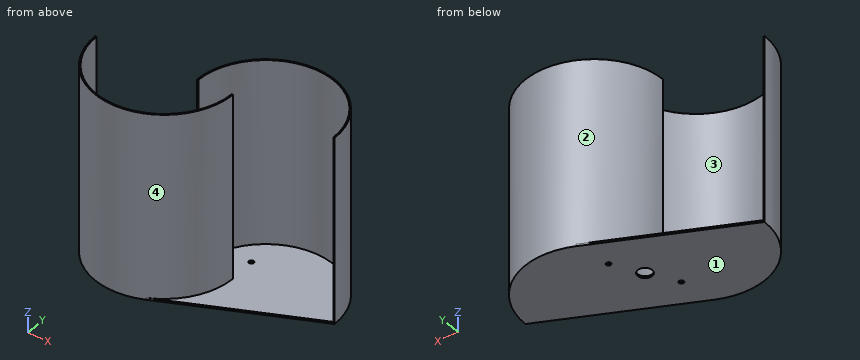
Autodesk Fusion 360 part; units mm, degrees
sketch "Turbine" plane through (0, 0, 0) normal (0, 0, 1) x (1, 0, 0) in component "Savonius Turbine"
  line L0 (10.5, 0) -> (-10.5, 0) construction
  arc A0 (74.2, 0) -> (-10.5, 0) centre (31.85, 0) ccw
  line L1 (31.85, 0) -> (74.2, 0) construction
  line L2 (31.85, 0) -> (-10.5, 0) construction
  arc A1 (-74.2, 0) -> (10.5, 0) centre (-31.85, 0) ccw
  line L3 (-31.85, 0) -> (-74.2, 0) construction
  line L4 (-31.85, 0) -> (10.5, 0) construction
  arc A2 (75, 0) -> (-11.3, 0) centre (31.85, 0) ccw
  arc A3 (-75, 0) -> (11.3, 0) centre (-31.85, 0) ccw
  line L5 (75, 0) -> (74.2, 0)
  line L6 (-75, 0) -> (-74.2, 0)
  line L7 (11.3, 0) -> (10.5, 0)
  line L8 (-10.5, 0) -> (-11.3, 0)
  line L9 (74.2, 0) -> (11.3, 0)
  line L10 (-11.3, 0) -> (-74.2, 0)
  dimension "d7" = 21
  dimension "d9" = 180
  dimension "d11" = 42.35
  dimension "d12" = 180
  dimension "d14" = 0.8
  dimension "d15" = 0.8
extrude "Extrude1" add sketch "Turbine" along normal blind 115.5 contours A0 A2 L5 L8 | A1 A3 L6 L7 makes body 1 at (-8.4391, -36.2471, 38.5) makes body 2 at (-4.9695, 22.4999, 38.5) in component "Savonius Turbine"
extrude "Extrude2" add sketch "Turbine" along normal blind 1.2 contours A0 A1 L7 L8 L9 L10 bodies 1 2 in component "Savonius Turbine"
sketch "Mounting Holes" plane through (0, 0, 0) normal (0, 0, 1) x (1, 0, 0) in component "Savonius Turbine"
  line L0 (-10.1657, -17.2238) -> (10.1657, 17.2238) construction
  circle A0 centre (-10.1657, -17.2238) radius 1.5
  circle A1 centre (10.1657, 17.2238) radius 1.5
  circle A2 centre (0, 0) radius 4.5
  dimension "d24" = 40
  dimension "d25" = 3
  dimension "d26" = 9
extrude "Extrude3" cut sketch "Mounting Holes" along normal through all bodies 1 in component "Savonius Turbine"
sketch "Base Reinforcement" plane through (0, 0, 0) normal (0, 0, 1) x (1, 0, 0) in component "Savonius Turbine"
  circle A0 centre (0, 0) radius 4.5
  circle A1 centre (-10.1657, -17.2238) radius 1.5
  circle A2 centre (10.1657, 17.2238) radius 1.5
  arc A3 (-75, 0) -> (11.3, 0) centre (-31.85, 0) ccw
  line L0 (-75, 0) -> (-11.3, 0)
  arc A4 (75, 0) -> (-11.3, 0) centre (31.85, 0) ccw
  line L1 (75, 0) -> (11.3, 0)
  line L2 (75, 0) -> (-14.4244, -39.475)
  line L3 (-75, 0) -> (14.4244, 39.475)
extrude "Extrude4" add sketch "Base Reinforcement" along normal blind 1.2 contours L0 A4 L3 | A3 L1 L2 bodies 1 in component "Savonius Turbine"
component "Savonius Turbine" placed x (1, 0, 0) y (0, 1, 0) z (0, 0, 1) at (0, 0, 0)
equation "Width = 150 mm"
equation "Height = Width * AspectRatio"
equation "Overlap = OverlapPercent * Width"
equation "BladeDiameter = ( Width + Overlap ) / 2 - BladeThickness"
equation "d7 = Overlap"
equation "d11 = BladeDiameter / 2"
equation "BladeThickness = 0.8 mm"
equation "d14 = BladeThickness"
equation "d15 = BladeThickness"
equation "d19 = Height"
equation "BaseThickness = 1.2 mm"
equation "d22 = BaseThickness"
equation "d28 = BaseThickness"
The listing builds one solid part. Answer for the finished solid, in the listing's coordinates (mm). Face numbers are marked on the shaded views. Give positions to 0.01 mm unless a question says otherwise; leave off trailing zeros. Order: outer loops, then holes, each group sorted by start corner. A loop starts at its lowest first (then second) coordinate and runs counter-clockwise, first axis right, second up. Notation, with made-up numbers: (30, 12) - (51, 12) arc R12 ccw to (51, 33) - close; hole circle Ø10 at (18.5, -40). An arc over 180 degrees is marked (long way). Use one line per item in the form item = value.
1) Find section B-B on x = 0. Determine the outline of the cut face in (y, z), and give its area (3 significant figures).
Verdict:
outline = (-33.11, 0) - (-4.5, 0) - (-4.5, 1.2) - (-27.91, 1.2) - (-27.91, 115.5) - (-29.11, 115.5) - (-29.11, 1.2) - (-33.11, 1.2) - close; (4.5, 0) - (33.11, 0) - (33.11, 1.2) - (29.11, 1.2) - (29.11, 115.5) - (27.91, 115.5) - (27.91, 1.2) - (4.5, 1.2) - close
area = 343 mm^2
2) Find section C-C on y = -37.5. Determine the outline of the cut face in (x, z).
Verdict:
outline = (-53.2, 0) - (-9.95, 0) - (-9.95, 1.2) - (-10.5, 1.2) - (-10.5, 115.5) - (-12.17, 115.5) - (-12.17, 1.2) - (-51.53, 1.2) - (-51.53, 115.5) - (-53.2, 115.5) - close
3) Each of these flat-tipped pins is pushed along its axis until it touches: pin 1 (8 mm diameter, centred on y = 28, z = 61.5, fed in from -X); pin 2 (0.6 mm diameter, centred on x = 11, z = 63, fed in from +Y); pin 3 (6 mm diameter, centred on x = -36.5, y = -29.5, fed in from +Z). Where does it stop, or does it pass through?
Verdict:
pin_1 = -4.01
pin_2 = 37.94
pin_3 = 1.2
4) Find section A-A on z = 67. Determine the outline of the cut face in (x, y).
Verdict:
outline = (-75, 0) arc R43.15 ccw to (11.3, 0) - (10.5, 0) arc R42.35 cw to (-74.2, 0) - close; (-11.3, 0) - (-10.5, 0) arc R42.35 cw to (74.2, 0) - (75, 0) arc R43.15 ccw to start
5) Find section D-D on x = 45.5. Determine the outline of the cut face in (y, z).
Verdict:
outline = (-13.02, 0) - (40.93, 0) - (40.93, 115.5) - (40.09, 115.5) - (40.09, 1.2) - (-13.02, 1.2) - close
6) The mould has two halves that part along Y. Classify the marked faces 1, 2, 3 and 4: released by +Y, released by -Y, zero draft, split by the parting line, or undercut.
Verdict:
face_1 = zero draft
face_2 = released by +Y
face_3 = undercut
face_4 = released by -Y
7) Consider probe 1 along X at (y, z) = (-1, 75.5); probe 2 along X at (y, z) = (0, 0.85); probe 3 along Z at (x, y) = (-17, -38). Determine where each line is inside the solid, lowest interval first. Write a range as [from, to].
Verdict:
probe_1 = [-74.99, -74.19], [10.49, 11.29]
probe_2 = [-75, -4.5], [4.5, 75]
probe_3 = [0, 1.2]
